Here's the drawing with two shaded views (mm, measured from the low corner). I have some questions. A direction names the side the tool comes from. Coordinates: 2 decimals unless noted, no trailing zeros. Loops run counter-clockwise (first coordinate to the right, second up) from the corner with the lowest first, then second, coordinate; pieces in that order, holes last. Notation, with made-up numbers: M 72.25,-29 L 114.25,-29 A19 cw 114.25,3 Z; hole C 49.5,8 d7. An arc over 180 degrees is marked long. Return JSON: item names as keys, results as strings. Group by question number.
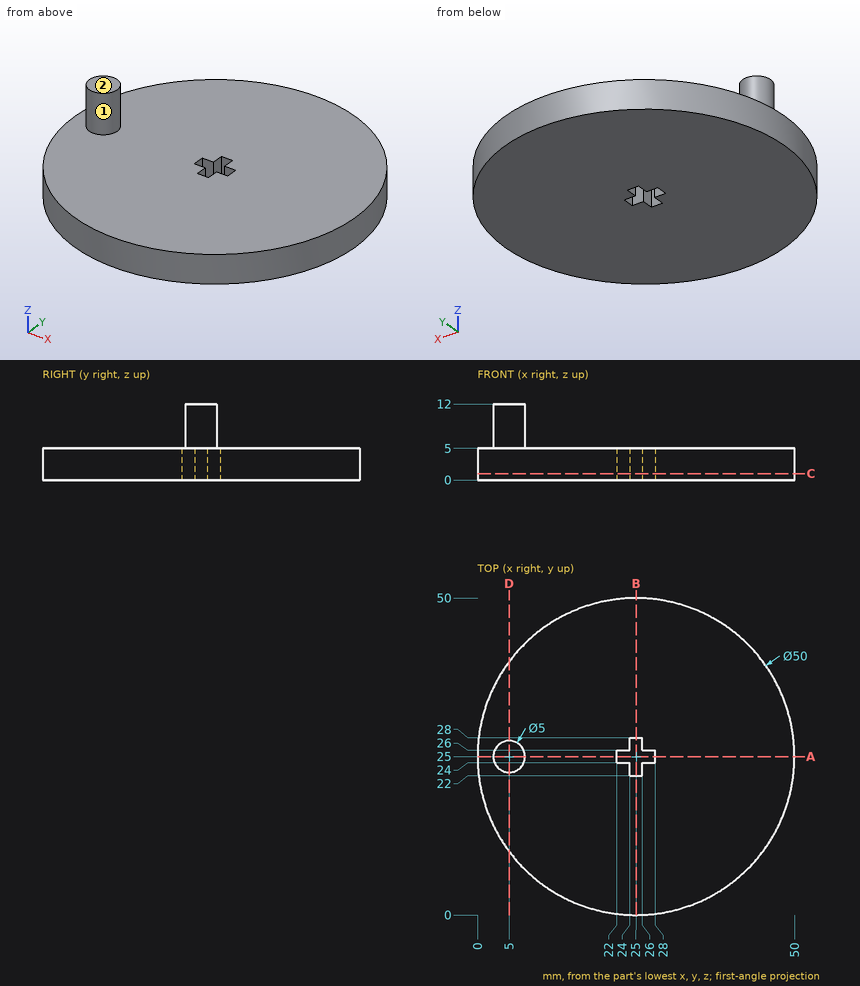
1) For pin 1 (0.6 mm diameter, centred on x = 25, z = 3, fed in from +Y); pin 2 (1.6 mm diameter, centred on x = 27, z = 1.5, fed in from -Y); pin 3 (1.6 mm diameter, centred on y = 23, z = 2.5, fed in from +X); pin 4 (5 mm diameter, centred on y = 9, z = 9.5, fed in from +X), each with a flat end and sliding along its axis, tell me the tip position at first contact or that it passes through.
2) Suppose I cut it at C-C, the plane z = 1. List the corners of the cut face in (x, y) for me.
3) Suppose I cut it at A-A, the plane y = 25. List the corners of the cut face in (x, z) for me.
4) For the marked faces 1 and 2, which set-ups out of +Z, -Z, +X, -X, +Y, -Y let a thin tool reach every point of the face, with its end or its side?
5) Suppose I cut it at D-D, the plane x = 5. List the corners of the cut face in (y, z) for me, then the cut area to 3 significant figures.
6) Suppose I cut it at B-B, the plane x = 25. List the corners of the cut face in (y, z) for me, then the cut area to 3 significant figures.
7) If I drill on line 1 (Z direction, x = 19, y = 25); line 2 (X direction, y = 24.5, z = 6); line 3 (Y direction, x = 6, z = 8), over which ranges is the centre line in solid material (lowest first)? Write a range as from..to.
Returned:
{
 "1": {"pin 1": "stops at y = 50", "pin 2": "stops at y = 0.03", "pin 3": "stops at x = 49.97", "pin 4": "passes through"},
 "2": {"outline": "C 25,25 d50; hole M 22,24 L 24,24 L 24,22 L 26,22 L 26,24 L 28,24 L 28,26 L 26,26 L 26,28 L 24,28 L 24,26 L 22,26 Z"},
 "3": {"outline": "M 0,0 L 22,0 L 22,5 L 7.5,5 L 7.5,12 L 2.5,12 L 2.5,5 L 0,5 Z; M 28,0 L 50,0 L 50,5 L 28,5 Z"},
 "4": {"face 1": "+Z", "face 2": "+Z, +X, -X, +Y, -Y"},
 "5": {"outline": "M 10,0 L 40,0 L 40,5 L 27.5,5 L 27.5,12 L 22.5,12 L 22.5,5 L 10,5 Z", "area": "185 mm²"},
 "6": {"outline": "M 0,0 L 22,0 L 22,5 L 0,5 Z; M 28,0 L 50,0 L 50,5 L 28,5 Z", "area": "220 mm²"},
 "7": {"line 1": "z = 0..5", "line 2": "x = 2.55..7.45", "line 3": "y = 22.71..27.29"}
}
